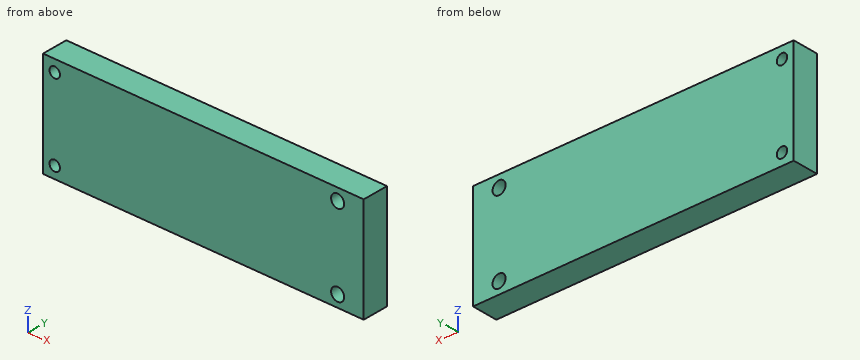
Autodesk Inventor part; units mm, degrees
ref_plane "YZ Plane" through (0, 0, 0) normal (1, 0, 0) x (0, 1, 0)
ref_plane "XZ Plane" through (0, 0, 0) normal (0, 1, 0) x (-1, 0, 0)
ref_plane "XY Plane" through (0, 0, 0) normal (0, 0, 1) x (1, 0, 0)
sketch "Skizze1" plane through (0, 0, 0) normal (0, 1, 0) x (-1, 0, 0)
  line L0 (0, 0) -> (59, 0)
  line L1 (59, 0) -> (59, -20)
  line L2 (59, -20) -> (0, -20)
  line L3 (0, -20) -> (0, 0)
  dimension "d0" = 59
  dimension "d1" = 20
extrude "Extrusion1" add sketch "Skizze1" along normal blind 5
sketch "Skizze2" plane through (0, 5, 0) normal (0, 1, 0) x (1, 0, 0)
  point P0 (0, 0)
sketch "Skizze3" plane through (0, 5, 0) normal (0, 1, 0) x (1, 0, 0)
  line L0 (0, 0) -> (0, 20)
  line L1 (0, 0) -> (-2.5, 0)
  line L2 (-59, 0) -> (0, 0)
  line L3 (-2.5, 0) -> (-2.5, 2.25)
  line L4 (-2.5, 2.25) -> (-2.5, 17.75)
  dimension "d4" = 2.5
  dimension "d5" = 2.25
  dimension "d6" = 15.5
hole "Bohrung1" at (-2.5, 5, -2.25) at (-2.5, 5, -17.75) direction (0, -1, 0) diameter 2.5 end through all
sketch "Skizze4" plane through (0, 5, 0) normal (0, 1, 0) x (1, 0, 0)
  line L0 (-59, 0) -> (0, 0)
  line L1 (-58.751, 0) -> (-56.751, 0)
  line L2 (-56.751, 0) -> (-59.001, 0)
  line L3 (-56.751, 0) -> (-56.751, 2.25)
  line L4 (-56.751, 2.25) -> (-56.751, 17.75)
  dimension "d14" = 2
  dimension "d16" = 2.25
  dimension "d17" = 15.5
hole "Bohrung2" at (-56.751, 5, -2.25) at (-56.751, 5, -17.75) direction (0, -1, 0) diameter 2 end through all
sketch "Skizze5" plane through (0, 0, 0) normal (1, 0, 0) x (0, 0, -1)
  line L0 (20, 0) -> (0, 0)
  line L1 (0, 0) -> (20, 0)
  line L2 (20, 0) -> (20, 5)
  line L3 (20, 5) -> (0, 5)
  line L4 (0, 5) -> (0, 0)
extrude "Extrusion2" add sketch "Skizze5" along normal blind 2.5
properties part number "Sensor_Halterung_Teil2ipt" material "Holz (Eiche)"
Model file for the job. Use its own axes, mm. Give positions to 0.01 mm unless a question says otherwise; leave off trailing zeros. Loops run counter-clockwise (first coordinate to the right, second up) from the corner with the lowest first, then second, coordinate; pieces in that order, holes last. Notation, with made-up numbers: M 71.5,84.5 L 129.5,84.5 A33 cw 129.5,122.5 Z; hole C -25.75,-10 d9. An arc over 180 degrees is marked long. Use one line per item in the form item = value.
Item 1: Drill centre lines: L1, parallel to X at y = 1.45, z = -17.75; L2, parallel to Z at x = -2.5, y = 1.2; L3, parallel to Z at x = -3, y = 2.4. Where is each one in solid material? Low to high.
Filled in:
L1 = -59 to -57.75, -55.75 to -3.75, -1.25 to 2.5
L2 = -20 to -19, -16.5 to -3.5, -1 to 0
L3 = -20 to -18.9, -16.6 to -3.4, -1.1 to 0
Item 2: Slice it at A-A on z = -2.25. List the corners of the cut face in (x, y), and give its area (3 significant figures).
Filled in:
outline = M -59,0 L -57.75,0 L -57.75,5 L -59,5 Z; M -55.75,0 L -3.75,0 L -3.75,5 L -55.75,5 Z; M -1.25,0 L 2.5,0 L 2.5,5 L -1.25,5 Z
area = 285 mm^2
Item 3: Flat gauge pin, fed straight in: pin 1 Ø10 at (x, z) = (-31.5, -14) entering from -Y. Where does the tip first touch, or does it go through?
Filled in:
pin_1 = 0
Item 4: Slice it at B-B on x = -2.5. List the corners of the cut face in (y, z).
Filled in:
outline = M 0,-20 L 5,-20 L 5,-19 L 0,-19 Z; M 0,-16.5 L 5,-16.5 L 5,-3.5 L 0,-3.5 Z; M 0,-1 L 5,-1 L 5,0 L 0,0 Z
